Part model, mm, in its own coordinate system. A direction names the side the tool comes from. Give positions to 0.01 mm unless a question says otherwise; leave off trailing zeros. Order: outer loops, then holes, each group sorted by start corner. A loop starts at its lowest first (then second) coordinate and runs counter-clockwise, first axis right, second up. Notation, with made-up numbers: (35, 47.25) -> (77, 47.25) arc R25 cw to (77, 76.25) -> close; hole circle Ø10 at (62.5, 80.5). An arc over 180 degrees is marked (long way). Write item = value, one per line. Start each with the question number.
(1) Probe line 1 along X through (y, z) = (3.75, 5.5); line 2 along X through (y, z) = (27.5, 6); line 3 along Y through (x, z) = (-6, -5.5). List the from-to ranges inside material, lowest first. Write a range as from..to.
(2) Saw through at C-C, the plane z = 14.5. List the corners of the cut face in (x, y).
(3) Saw through at B-B, the plane y = 20.5. List the corners of the cut face in (x, z), then the cut area to 3 significant figures.
(4) Saw through at D-D, the plane x = 0. State how many separate pieces and enclosed holes the cut face has, then the cut area to 3 significant figures.
(5) Which spindle directions (+Z, -Z, +X, -X, +Y, -Y) get a long thin tool onto all of the face, cutting with end or side? Do faces 5 (the flat face through (0, 21, -14.5)), 6 (the cylindrical face through (-3.905, 36.528, -0.867)), 7 (the cylindrical face through (-1.05, 36.08, -13.54)), 8 (the cylindrical face through (8.107, 39.627, 6.238)). Say none if no direction does.
(6) Two-plate mould, pull along X, no slides. Class faces 1 (the flat face through (8, 37.7, -7)), 2 (the flat face through (-20, 20, 0)), 3 (the flat face through (17, 21, 10)), 4 (the flat face through (0, 7, -18)): pulls with the +X half, pulls with the -X half, needs draft (parallel to the pull), parting line crosses it, or undercut.
(7) Saw through at A-A, the plane z = -21.5. List the corners of the cut face in (x, y).
(8) Flat gauge pins, fed straight in: pin 1 (2.5 mm diameter, centred on x = 0, z = -21.5, fed in from -Y); pin 2 (8 mm diameter, centred on x = -13.5, y = 12, fed in from -Z); pin 3 (14 mm diameter, centred on x = 3.5, y = 15.5, fed in from +Z); pin 4 (5 mm diameter, centred on x = 14, y = 37, fed in from +Z). Where does each tip first touch, or does it go through?
from build123d import *

# Parameters (mm, degrees)
SKETCH1_W           = 40
SKETCH1_H           = 35
BOSS_EXTRUDE1_DEPTH = 7
BOSS_EXTRUDE2_DEPTH = 27.5
SKETCH3_W           = 40
SKETCH3_H           = 35
BOSS_EXTRUDE3_DEPTH = 7
SKETCH4_R           = 1.6
SKETCH4_R_2         = 4
CUT_EXTRUDE1_DEPTH  = 57
SKETCH5_R           = 2.75
CUT_EXTRUDE2_DEPTH  = 3.2
SKETCH6_R           = 8.25
CUT_EXTRUDE3_DEPTH  = 3
SKETCH7_W           = 4
SKETCH7_H           = 27.5
CUT_EXTRUDE4_DEPTH  = 12.4
SKETCH8_W           = 40
SKETCH8_H           = 8
SKETCH8_R           = 1.65
BOSS_EXTRUDE4_DEPTH = 7
SKETCH10_R          = 2.75
CUT_EXTRUDE5_DEPTH  = 3.2
BOSS_EXTRUDE5_START = -7
SKETCH11_R          = 4
BOSS_EXTRUDE5_DEPTH = 7


with BuildPart() as part:
    # Sketch1 → Boss-Extrude1 (new body)
    with BuildSketch(Plane(origin=(0, 0, 0), x_dir=(1, 0, 0), z_dir=(0, 1, 0))):
        Rectangle(SKETCH1_W, SKETCH1_H)
    extrude(amount=BOSS_EXTRUDE1_DEPTH)

    # Sketch2 → Boss-Extrude2 (add)
    with BuildSketch(Plane(origin=(0, 7, 0), x_dir=(1, 0, 0), z_dir=(0, 1, 0))):
        Polygon((-20, -17.5), (-17, -17.5), (-17, 14.5), (17, 14.5), (17, -17.5), (20, -17.5), (20, 17.5), (-20, 17.5), align=None)
    extrude(amount=BOSS_EXTRUDE2_DEPTH)

    # Sketch3 → Boss-Extrude3 (add)
    with BuildSketch(Plane(origin=(0, 34.5, 0), x_dir=(1, 0, 0), z_dir=(0, 1, 0))):
        Rectangle(SKETCH3_W, SKETCH3_H)
    extrude(amount=BOSS_EXTRUDE3_DEPTH)

    # Sketch4 → Cut-Extrude1 (cut)
    with BuildSketch(Plane(origin=(0, 41.5, 0), x_dir=(1, 0, 0), z_dir=(0, 1, 0))):
        with Locations(Location((0, 11, 0), (0, 0, 270))):
            Circle(SKETCH4_R)
        with Locations(Location((9.526279442, 5.5, 0), (0, 0, 270))):
            Circle(SKETCH4_R)
        with Locations(Location((9.526279442, -5.5, 0), (0, 0, 270))):
            Circle(SKETCH4_R)
        with Locations(Location((0, -11, 0), (0, 0, 270))):
            Circle(SKETCH4_R)
        with Locations(Location((-9.526279442, -5.5, 0), (0, 0, 270))):
            Circle(SKETCH4_R)
        with Locations(Location((-9.526279442, 5.5, 0), (0, 0, 270))):
            Circle(SKETCH4_R)
        with Locations(Location((0, 0, 0), (0, 0, 270))):
            Circle(SKETCH4_R_2)
    extrude(amount=-CUT_EXTRUDE1_DEPTH, mode=Mode.SUBTRACT)

    # Sketch5 → Cut-Extrude2 (cut)
    with BuildSketch(Plane.XZ.offset(-34.5)):
        with Locations(Location((0, 11, 0), (0, 0, 270))):
            Circle(SKETCH5_R)
        with Locations(Location((0, -11, 0), (0, 0, 270))):
            Circle(SKETCH5_R)
        with Locations(Location((9.526279442, -5.5, 0), (0, 0, 270))):
            Circle(SKETCH5_R)
        with Locations(Location((9.526279442, 5.5, 0), (0, 0, 270))):
            Circle(SKETCH5_R)
        with Locations(Location((-9.526279442, 5.5, 0), (0, 0, 270))):
            Circle(SKETCH5_R)
        with Locations(Location((-9.526279442, -5.5, 0), (0, 0, 270))):
            Circle(SKETCH5_R)
    extrude(amount=-CUT_EXTRUDE2_DEPTH, mode=Mode.SUBTRACT)

    # Sketch6 → Cut-Extrude3 (cut)
    with BuildSketch(Plane(origin=(0, 41.5, 0), x_dir=(1, 0, 0), z_dir=(0, 1, 0))):
        with Locations(Location((0, 0, 0), (0, 0, 270))):
            Circle(SKETCH6_R)
    extrude(amount=-CUT_EXTRUDE3_DEPTH, mode=Mode.SUBTRACT)

    # Sketch7 → Cut-Extrude4 (cut)
    with BuildSketch(Plane(origin=(20, 0, 0), x_dir=(0, 0, -1), z_dir=(1, 0, 0))):
        with Locations((0, 20.75)):
            Rectangle(SKETCH7_W, SKETCH7_H)
    extrude(amount=-CUT_EXTRUDE4_DEPTH, mode=Mode.SUBTRACT)

    # Sketch8 → Boss-Extrude4 (add)
    # profile 1 of 2: a face of its own
    with BuildSketch(Plane(origin=(0, 0, 0), x_dir=(1, 0, 0), z_dir=(0, 1, 0))):
        with Locations((0, -21.5)):
            Rectangle(SKETCH8_W, SKETCH8_H)
        with Locations(Location((0, -21.5, 0), (0, 0, 90))):
            Circle(SKETCH8_R, mode=Mode.SUBTRACT)
    # profile 2 of 2: a face of its own
    with BuildSketch(Plane(origin=(0, 0, 0), x_dir=(1, 0, 0), z_dir=(0, 1, 0))):
        with Locations((0, 21.5)):
            Rectangle(SKETCH8_W, SKETCH8_H)
        with Locations(Location((0, 21.5, 0), (0, 0, 90))):
            Circle(SKETCH8_R, mode=Mode.SUBTRACT)
    extrude(amount=BOSS_EXTRUDE4_DEPTH)

    # Sketch10 → Cut-Extrude5 (cut)
    with BuildSketch(Plane(origin=(0, 7, 0), x_dir=(1, 0, 0), z_dir=(0, 1, 0))):
        with Locations(Location((0, 21.5, 0), (0, 0, 270))):
            Circle(SKETCH10_R)
        with Locations(Location((0, -21.5, 0), (0, 0, 270))):
            Circle(SKETCH10_R)
    extrude(amount=-CUT_EXTRUDE5_DEPTH, mode=Mode.SUBTRACT)

    # Sketch11 → Boss-Extrude5 (add)
    with BuildSketch(Plane.XZ.offset(BOSS_EXTRUDE5_START)):
        with Locations(Location((0, 0, 0), (0, 0, 90))):
            Circle(SKETCH11_R)
    extrude(amount=BOSS_EXTRUDE5_DEPTH)


solid = part.part
Results list:
q1.line_1 = -20..-11.13, -7.93..7.93, 11.13..20
q1.line_2 = -20..-17, 17..20
q1.line_3 = 0..7, 34.5..38.5
q2.outline = (-20, 0) -> (20, 0) -> (20, 41.5) -> (-20, 41.5) -> close; hole (-17, 7) -> (17, 7) -> (17, 34.5) -> (-17, 34.5) -> close
q3.outline = (-20, -17.5) -> (20, -17.5) -> (20, -2) -> (17, -2) -> (17, -14.5) -> (-17, -14.5) -> (-17, 17.5) -> (-20, 17.5) -> close; (17, 2) -> (20, 2) -> (20, 17.5) -> (17, 17.5) -> close
q3.area = 300 mm^2
q4.separate_pieces = 8
q4.enclosed_holes = 0
q4.area = 438 mm^2
q5.face_5 = +Z
q5.face_6 = +Y
q5.face_7 = none
q5.face_8 = +Y, -Y
q6.face_1 = undercut
q6.face_2 = pulls with the -X half
q6.face_3 = undercut
q6.face_4 = needs draft
q7.outline = (-20, 0) -> (-1.65, 0) -> (-1.65, 3.8) -> (-2.75, 3.8) -> (-2.75, 7) -> (-20, 7) -> close; (1.65, 0) -> (20, 0) -> (20, 7) -> (2.75, 7) -> (2.75, 3.8) -> (1.65, 3.8) -> close
q8.pin_1 = through
q8.pin_2 = -17.5
q8.pin_3 = -14.5
q8.pin_4 = 17.5
